from build123d import *

# Parameters (mm, degrees)
SKETCH1_R             = 193.675
SKETCH1_R_2           = 174.625
BOSS_EXTRUDE1_DEPTH   = 3.175
SKETCH1_R_3           = 33.3375
BOSS_EXTRUDE1_2_DEPTH = 3.175
BOSS_EXTRUDE2_START   = -3.175
BOSS_EXTRUDE2_DEPTH   = 3.175
SKETCH3_R             = 2.15265
CUT_EXTRUDE1_DEPTH    = 3.175
SKETCH4_R             = 2.15265
CUT_EXTRUDE2_DEPTH    = 3.175
CIRPATTERN1_COUNT     = 6


with BuildPart() as part:
    # Sketch1 → Boss-Extrude1 (new body)
    with BuildSketch(Plane.XY):
        Circle(SKETCH1_R)
        Circle(SKETCH1_R_2, mode=Mode.SUBTRACT)
    extrude(amount=BOSS_EXTRUDE1_DEPTH)



with BuildPart() as body_2:
    # Sketch1 → Boss-Extrude1 2 (new body)
    with BuildSketch(Plane.XY):
        Circle(SKETCH1_R_3)
        Polygon((7.332348419, 0), (3.666174209, 6.35), (-3.666174209, 6.35), (-7.332348419, 0), (-3.666174209, -6.35), (3.666174209, -6.35), align=None, mode=Mode.SUBTRACT)
    extrude(amount=BOSS_EXTRUDE1_2_DEPTH)


with BuildPart() as part_1:
    add(part.part)

    add(body_2.part)  # Boss-Extrude2 merges body 2
    # Sketch2 → Boss-Extrude2 (add)
    with BuildSketch(Plane.XY.offset(3.175).offset(BOSS_EXTRUDE2_START)):
        with BuildLine():
            Line((15.875, 49.493351826), (15.875, 159.383735055))
            ThreePointArc((15.875, 159.383735055), (20.425550361, 169.124190413), (30.816176471, 171.884420157))
            ThreePointArc((30.816176471, 171.884420157), (0, 174.625), (-30.816176471, 171.884420157))
            ThreePointArc((-30.816176471, 171.884420157), (-20.425550361, 169.124190413), (-15.875, 159.383735055))
            Line((-15.875, 159.383735055), (-15.875, 49.493351826))
            ThreePointArc((-15.875, 49.493351826), (-22.225, 38.494829198), (-34.925, 38.494829198))
            Line((-34.925, 38.494829198), (-130.092863507, 93.440020812))
            ThreePointArc((-130.092863507, 93.440020812), (-136.253070112, 102.251140706), (-133.448186135, 112.62980175))
            ThreePointArc((-133.448186135, 112.62980175), (-151.229686136, 87.3125), (-164.264362606, 59.254618408))
            ThreePointArc((-164.264362606, 59.254618408), (-156.678620473, 66.873049707), (-145.967863507, 65.943714242))
            Line((-145.967863507, 65.943714242), (-50.8, 10.998522628))
            ThreePointArc((-50.8, 10.998522628), (-44.45, 0), (-50.8, -10.998522628))
            Line((-50.8, -10.998522628), (-145.967863507, -65.943714242))
            ThreePointArc((-145.967863507, -65.943714242), (-156.678620473, -66.873049707), (-164.264362606, -59.254618408))
            ThreePointArc((-164.264362606, -59.254618408), (-151.229686136, -87.3125), (-133.448186135, -112.62980175))
            ThreePointArc((-133.448186135, -112.62980175), (-136.253070112, -102.251140706), (-130.092863507, -93.440020812))
            Line((-130.092863507, -93.440020812), (-34.925, -38.494829198))
            ThreePointArc((-34.925, -38.494829198), (-22.225, -38.494829198), (-15.875, -49.493351826))
            Line((-15.875, -49.493351826), (-15.875, -159.383735055))
            ThreePointArc((-15.875, -159.383735055), (-20.425550361, -169.124190413), (-30.816176471, -171.884420157))
            ThreePointArc((-30.816176471, -171.884420157), (0, -174.625), (30.816176471, -171.884420157))
            ThreePointArc((30.816176471, -171.884420157), (20.425550361, -169.124190413), (15.875, -159.383735055))
            Line((15.875, -159.383735055), (15.875, -49.493351826))
            ThreePointArc((15.875, -49.493351826), (22.225, -38.494829198), (34.925, -38.494829198))
            Line((34.925, -38.494829198), (130.092863507, -93.440020812))
            ThreePointArc((130.092863507, -93.440020812), (136.253070112, -102.251140706), (133.448186135, -112.62980175))
            ThreePointArc((133.448186135, -112.62980175), (151.229686136, -87.3125), (164.264362606, -59.254618408))
            ThreePointArc((164.264362606, -59.254618408), (156.678620473, -66.873049707), (145.967863507, -65.943714242))
            Line((145.967863507, -65.943714242), (50.8, -10.998522628))
            ThreePointArc((50.8, -10.998522628), (44.45, 0), (50.8, 10.998522628))
            Line((50.8, 10.998522628), (145.967863507, 65.943714242))
            ThreePointArc((145.967863507, 65.943714242), (156.678620473, 66.873049707), (164.264362606, 59.254618408))
            ThreePointArc((164.264362606, 59.254618408), (151.229686136, 87.3125), (133.448186135, 112.62980175))
            ThreePointArc((133.448186135, 112.62980175), (136.253070112, 102.251140706), (130.092863507, 93.440020812))
            Line((130.092863507, 93.440020812), (34.925, 38.494829198))
            ThreePointArc((34.925, 38.494829198), (22.225, 38.494829198), (15.875, 49.493351826))
        make_face()
        Polygon((7.332348419, 0), (3.666174209, 6.35), (-3.666174209, 6.35), (-7.332348419, 0), (-3.666174209, -6.35), (3.666174209, -6.35), align=None, mode=Mode.SUBTRACT)
    extrude(amount=BOSS_EXTRUDE2_DEPTH)

    # Sketch3 → Cut-Extrude1 (cut)
    with BuildSketch(Plane.XY.offset(3.175)):
        with Locations((0, 38.1)):
            Circle(SKETCH3_R)
        with Locations((32.995567884, 19.05)):
            Circle(SKETCH3_R)
        with Locations((32.995567884, -19.05)):
            Circle(SKETCH3_R)
        with Locations((0, -38.1)):
            Circle(SKETCH3_R)
        with Locations((-32.995567884, -19.05)):
            Circle(SKETCH3_R)
        with Locations((-32.995567884, 19.05)):
            Circle(SKETCH3_R)
    extrude(amount=-CUT_EXTRUDE1_DEPTH, mode=Mode.SUBTRACT)

    # Sketch4 → Cut-Extrude2 (cut)
    with BuildSketch(Plane.XY.offset(3.175)):
        with Locations((-9.520641414, 181.519243783)):
            Circle(SKETCH4_R)
        with Locations((9.520641414, 181.519243783)):
            Circle(SKETCH4_R)
    cut_extrude2 = extrude(amount=-CUT_EXTRUDE2_DEPTH, mode=Mode.SUBTRACT)

    # CirPattern1: Cut-Extrude2 ×6 about axis
    cirpattern1_axis = Axis((0, 0, 0), (0, 0, 1))
    for i in range(1, CIRPATTERN1_COUNT):
        add(cut_extrude2.rotate(cirpattern1_axis, i * 360 / CIRPATTERN1_COUNT), mode=Mode.SUBTRACT)


solid = part_1.part
Design review of the part built by this model. Coordinates are the model's own, in mm. A direction names the side the tool comes from. Give positions to 0.01 mm unless a question says otherwise; leave off trailing zeros. Loops run counter-clockwise (first coordinate to the right, second up) from the corner with the lowest first, then second, coordinate; pieces in that order, holes last. Notation, with made-up numbers: (-21, -18.5) -> (11, -18.5) arc R12 cw to (11, -9.5) -> close; hole circle Ø8 at (19.5, 23). An arc over 180 degrees is marked (long way). One line per question, with ' | ' between items. Start each with the question number.
(1) We need section B-B (y = 128). State the section outline as (x, z) points (3 decimals).
(2) For faces 4 (the face through (-3, -40, 3.175)), 5 (the face through (22.06, -38.59, 1.57)), list the 3-axis set-ups (+Z, -Z, +X, -X, +Y, -Y) from which the entire face can be reached by the end or side of a thin tool; tool diameter is ignored.
(3) For line 1 (X direction, y = -22, z = 1.3); line 2 (X direction, y = 4, z = 1.1); line 3 (X direction, y = 140, z = 1.5) (3 decimals), list the stretches that pass through material, from the lowest coordinate up.
(4) We need section C-C (x = 26). State the section outline as (y, z) points (3 decimals), and give its area (3 significant figures).
(5) We need section D-D (z = 2.5). State how many separate pieces and enclosed holes the cut face has, and give its area (3 significant figures).
(6) Insertion check: P1, Ø2, axis at x = -67.5, y = -35, coming from the -Z side; P2, Ø1.5, axis at y = 128, z = 1, coming from the +X side. Each pin has a flat end and moves straight along its axis. Give the tip position at first contact, or say it passes through.
(7) We need section A-A (x = 68.5). State the section outline as (y, z) points (3 decimals).
(8) Draft analysis for pull direction X (two halves, no side actions). For faces 1 (the face through (-41.98, -189.07, 1.57)), 2 (the face through (-97.72, -38.09, 1.57)), 3 (the face through (-3, -40, 0)), state which applies: +X half, -X half, draft (parallel to the pull), parting line (faces both ways), or undercut.
The answers:
1) outline: (-145.348, 0) -> (-118.785, 0) -> (-118.785, 3.175) -> (-145.348, 3.175) -> close; (-15.875, 0) -> (15.875, 0) -> (15.875, 3.175) -> (-15.875, 3.175) -> close; (118.785, 0) -> (145.348, 0) -> (145.348, 3.175) -> (118.785, 3.175) -> close
2) face 4: +Z, +X, -X, +Y, -Y | face 5: +Z, -Z
3) line 1: x = -192.42 to -173.23, -69.86 to 69.86, 173.23 to 192.42 | line 2: x = -193.63 to -174.58, -45.1 to -5.02, 5.02 to 45.1, 174.58 to 193.63 | line 3: x = -133.828 to -104.374, -15.875 to 15.875, 104.374 to 133.828
4) outline: (-191.922, 0) -> (-171.82, 0) -> (-171.82, 3.175) -> (-191.922, 3.175) -> close; (-37.057, 0) -> (37.057, 0) -> (37.057, 3.175) -> (-37.057, 3.175) -> close; (171.82, 0) -> (191.922, 0) -> (191.922, 3.175) -> (171.82, 3.175) -> close | area: 363 mm^2
5) separate pieces: 1 | enclosed holes: 25 | area: 53,500 mm^2
6) P1: stops at z = 0 | P2: stops at x = 146
7) outline: (-181.157, 0) -> (-160.629, 0) -> (-160.629, 3.175) -> (-181.157, 3.175) -> close; (-57.879, 0) -> (-21.218, 0) -> (-21.218, 3.175) -> (-57.879, 3.175) -> close; (21.218, 0) -> (57.879, 0) -> (57.879, 3.175) -> (21.218, 3.175) -> close; (160.629, 0) -> (181.157, 0) -> (181.157, 3.175) -> (160.629, 3.175) -> close
8) face 1: parting line | face 2: undercut | face 3: draft
